```python
from build123d import *

# Parameters (mm, degrees)
SKETCH1_R           = 29.55
BOSS_EXTRUDE1_DEPTH = 61.5
SKETCH2_R           = 28.2
CUT_EXTRUDE1_DEPTH  = 61.5
CUT_EXTRUDE2_START  = -2.5
CUT_EXTRUDE2_DEPTH  = 2.5


with BuildPart() as part:
    # Sketch1 → Boss-Extrude1 (new body)
    with BuildSketch(Plane(origin=(0, 0, 0), x_dir=(1, 0, 0), z_dir=(0, 1, 0))):
        with Locations(Location((0, 0, 0), (0, 0, 270))):
            Circle(SKETCH1_R)
    extrude(amount=BOSS_EXTRUDE1_DEPTH)

    # Sketch2 → Cut-Extrude1 (cut)
    with BuildSketch(Plane(origin=(0, 61.5, 0), x_dir=(1, 0, 0), z_dir=(0, 1, 0))):
        with Locations(Location((0, 0, 0), (0, 0, 270))):
            Circle(SKETCH2_R)
    extrude(amount=-CUT_EXTRUDE1_DEPTH, mode=Mode.SUBTRACT)

    # Sketch3 → Cut-Extrude2 (cut)
    with BuildSketch(Plane(origin=(0, 54.50000003, 0), x_dir=(1, 0, 0), z_dir=(0, 1, 0)).offset(CUT_EXTRUDE2_START)):
        with BuildLine():
            Line((-12.25, 26.891262521), (12.25, 26.891262521))
            ThreePointArc((12.25, 26.891262521), (0, 29.55), (-12.25, 26.891262521))
        make_face()
        with BuildLine():
            Line((26.891262521, 12.25), (26.891262521, -12.25))
            ThreePointArc((26.891262521, -12.25), (29.55, 0), (26.891262521, 12.25))
        make_face()
        with BuildLine():
            Line((12.25, -26.891262521), (-12.25, -26.891262521))
            ThreePointArc((-12.25, -26.891262521), (0, -29.55), (12.25, -26.891262521))
        make_face()
        with BuildLine():
            Line((-26.891262521, -12.25), (-26.891262521, 12.25))
            ThreePointArc((-26.891262521, 12.25), (-29.55, 0), (-26.891262521, -12.25))
        make_face()
    extrude(amount=CUT_EXTRUDE2_DEPTH, mode=Mode.SUBTRACT)


solid = part.part
```
Geometry: final body of the model. Coordinates: model frame, mm. A direction names the side the tool comes from. Coordinates: 2 decimals unless noted, no trailing zeros. Loops run counter-clockwise (first coordinate to the right, second up) from the corner with the lowest first, then second, coordinate; pieces in that order, holes last. Notation, with made-up numbers: M -1.5,-20.5 L 37.5,-20.5 A11 cw 37.5,-10.5 Z; hole C -23,4.25 d10. An arc over 180 degrees is marked long. Put each result on its own line as item: value.
(1) Access query for faces 3 (the face through (26.891, 53, -10)), 4 (the face through (10, 53, 26.891)), 5 (the face through (10, 53, -26.891)), 6 (the face through (-26.891, 53, 10)). Directions: +Z, -Z, +X, -X, +Y, -Y. A direction counts if a zero-diameter tool reaches every point of the face in a straight line with its end or side. Return the directions, or none.
Answer sheet:
face 3: +Z, -Z, +X
face 4: +Z, +X, -X
face 5: -Z, +X, -X
face 6: +Z, -Z, -X
(2) Cut plane A-A on z = 0. Return the cut outline in (x, y), then the cut area to 3 significant figures.
Answer sheet:
outline: M -29.55,0 L -28.2,0 L -28.2,52 L -29.55,52 Z; M -29.55,54.5 L -28.2,54.5 L -28.2,61.5 L -29.55,61.5 Z; M 28.2,0 L 29.55,0 L 29.55,52 L 28.2,52 Z; M 28.2,54.5 L 29.55,54.5 L 29.55,61.5 L 28.2,61.5 Z
area: 159 mm^2
(3) Cut plane C-C on z = -20. Return the cut outline in (x, y), then the cut area to 3 significant figures.
Answer sheet:
outline: M -21.75,0 L -19.88,0 L -19.88,61.5 L -21.75,61.5 Z; M 19.88,0 L 21.75,0 L 21.75,61.5 L 19.88,61.5 Z
area: 230 mm^2
(4) Material intervals for probe 1 along X at (y, z) = (39.5, 0); probe 2 along X at (y, z) = (35.5, 9), sorted ascending.
Answer sheet:
probe 1: x = -29.55 to -28.2, 28.2 to 29.55
probe 2: x = -28.15 to -26.73, 26.73 to 28.15
(5) First-contact query: pin 1 (3 mm diameter, centred on x = 20, y = 18, fed in from -Z); pin 2 (1.2 mm diameter, centred on y = 53, z = -10.5, fed in from +X); pin 3 (0.8 mm diameter, centred on x = 3, z = 27.5, fed in from -Y); pin 4 (2 mm diameter, centred on y = 29.5, z = -12, fed in from -X). Flat tips, straight axial feed; report the tip coordinate or a pass-through.
Answer sheet:
pin 1: stops at z = -23.04
pin 2: stops at x = 26.89
pin 3: passes through
pin 4: stops at x = -27.43
(6) Draft query along Y for faces 1 (the face through (-0.2, 54.5, 28.5)), 2 (the face through (26.891, 53, 10)). Return one class per face: pulls with the +Y half, pulls with the -Y half, needs draft (parallel to the pull), parting line crosses it, or undercut.
Answer sheet:
face 1: undercut
face 2: undercut
(7) Cut plane B-B on x = 0. Return the cut outline in (y, z).
Answer sheet:
outline: M 0,-29.55 L 52,-29.55 L 52,-28.2 L 0,-28.2 Z; M 0,28.2 L 52,28.2 L 52,29.55 L 0,29.55 Z; M 54.5,-29.55 L 61.5,-29.55 L 61.5,-28.2 L 54.5,-28.2 Z; M 54.5,28.2 L 61.5,28.2 L 61.5,29.55 L 54.5,29.55 Z
(8) Cut plane D-D on x = -18. Return the cut outline in (y, z), then the cut area to 3 significant figures.
Answer sheet:
outline: M 0,-23.44 L 61.5,-23.44 L 61.5,-21.71 L 0,-21.71 Z; M 0,21.71 L 61.5,21.71 L 61.5,23.44 L 0,23.44 Z
area: 212 mm^2
